Geometry check sheet. Reference: the model listing, model coordinates, mm. Give positions to 0.01 mm unless a question says otherwise; leave off trailing zeros. Write each loop counter-clockwise with the first axis right and the second up, starting at its lowest first coordinate (ties: lowest second). Pieces come first, ordered by that corner, then holes. Notation, with made-up numbers: M 67,61 L 104,61 A21 cw 104,91 Z; hole C -27.75,40 d10. An arc over 180 degrees is marked long. One line per item, written item: value. Start each with the question number.
1. Gauge pin test, flat end, axial feed: pin 1 (1 mm diameter, centred on x = 3, z = 232, fed in from -Y). Record the tip position at first contact, or that the pin passes through.
2. Cross-section at B-B on z = 241.5. Record the cut outline in (x, y), then the cut area to 3 significant figures.
3. Cross-section at A-A on x = 2.25. Count the separate pieces of the cut face and the enclosed holes in it, then the cut area to 3 significant figures.
4. Scan lines: line 1 (X direction, y = 5.7, z = 110); line 2 (Y direction, x = 6, z = 97); line 3 (Y direction, x = 1, z = 12). Record each from-to range of solid material in increasing order.
from build123d import *

# Parameters (mm, degrees)
SKETCH_W     = 11.4
SKETCH_H     = 11.4
SKETCH_R     = 1.5
PAD_DEPTH    = 275.2
SKETCH001_R  = 1.5
POCKET_DEPTH = 11.401


with BuildPart() as part:
    # Sketch → Pad (new body)
    with BuildSketch(Plane.XY):
        with Locations((5.7, 5.7)):
            Rectangle(SKETCH_W, SKETCH_H)
        with Locations((5.7, 5.7)):
            Circle(SKETCH_R, mode=Mode.SUBTRACT)
    extrude(amount=PAD_DEPTH)

    # Sketch001 → Pocket (cut, through all)
    with BuildSketch(Plane.YZ.offset(11.4)):
        with Locations((5.7, 142.35)):
            Circle(SKETCH001_R)
        with Locations((5.7, 134.35)):
            Circle(SKETCH001_R)
        with Locations((5.7, 19)):
            Circle(SKETCH001_R)
        with Locations((5.7, 11)):
            Circle(SKETCH001_R)
        with Locations((5.7, 89.35)):
            Circle(SKETCH001_R)
        with Locations((5.7, 81.35)):
            Circle(SKETCH001_R)
        with Locations((5.7, 185.65)):
            Circle(SKETCH001_R)
        with Locations((5.7, 177.65)):
            Circle(SKETCH001_R)
        with Locations((5.7, 264.2)):
            Circle(SKETCH001_R)
        with Locations((5.7, 256.2)):
            Circle(SKETCH001_R)
    extrude(amount=-POCKET_DEPTH, mode=Mode.SUBTRACT)


solid = part.part
Report:
1. pin 1: stops at y = 0
2. outline: M 0,0 L 11.4,0 L 11.4,11.4 L 0,11.4 Z; hole C 5.7,5.7 d3
2. area: 123 mm^2
3. separate pieces: 1
3. enclosed holes: 10
3. area: 3,070 mm^2
4. line 1: x = 0 to 4.2, 7.2 to 11.4
4. line 2: y = 0 to 4.23, 7.17 to 11.4
4. line 3: y = 0 to 4.58, 6.82 to 11.4
